Autodesk Inventor part; units mm, degrees
ref_plane "YZ Plane" through (0, 0, 0) normal (1, 0, 0) x (0, 1, 0)
ref_plane "XZ Plane" through (0, 0, 0) normal (0, 1, 0) x (-1, 0, 0)
ref_plane "XY Plane" through (0, 0, 0) normal (0, 0, 1) x (1, 0, 0)
sketch "Sketch1" plane through (0, 0, 0) normal (0, 1, 0) x (-1, 0, 0)
  line L0 (0, 0) -> (50, 0)
  line L1 (50, 0) -> (50, -50)
  line L2 (50, -50) -> (0, -50)
  line L3 (0, -50) -> (0, 0)
  dimension "d0" = 50
  dimension "d1" = 50
extrude "Extrusion1" add sketch "Sketch1" along normal blind 20
sketch "Sketch2" plane through (0, 0, 0) normal (1, 0, 0) x (0, 0, -1)
  line L0 (0, 20) -> (50, 20)
  line L1 (0, 0) -> (0, 20)
  line L2 (50, 0) -> (50, 20)
  point P0 (10, 10)
  point P1 (40, 10)
  dimension "d4" = 10
  dimension "d5" = 10
  dimension "d6" = 10
  dimension "d7" = 10
hole "Hole1" at (0, 10, -10) at (0, 10, -40) direction (-1, 0, 0) diameter 12 depth 50 tip angle 118
sketch "Sketch3" plane through (0, 20, 0) normal (0, 1, 0) x (1, 0, 0)
  line L0 (-50, 0) -> (-50, 50)
  line L1 (0, 50) -> (-50, 50)
  point P0 (0, 0)
  point P1 (-25, 25)
  dimension "d15" = 25
  dimension "d16" = 25
hole "Hole2" at (-25, 20, -25) direction (0, -1, 0) diameter 12 depth 50 tip angle 118
properties part number "Extruder mount top"
Check sheet for the modelled part. Datum: model origin and axes. Units: mm. Give positions to 0.01 mm unless a question says otherwise; leave off trailing zeros. Write each loop counter-clockwise with the first axis right and the second up, starting at its lowest first coordinate (ties: lowest second). Pieces come first, ordered by that corner, then holes.
Item 1: Cross-section at D-D (y = 1.5). Enter the section's corners in (x, z).
Item 2: Cross-section at B-B (y = 10). Enter the section's corners in (x, z), and give its area (3 significant figures).
Item 3: Scan lines: L1, parallel to Z at x = -34, y = 10; L2, parallel to Y at x = -21, z = -10; L3, parallel to Z at x = -25, y = 13. Record each from-to range of solid material in increasing order.
Item 4: Cross-section at A-A (z = -40). Enter the section's corners in (x, y), and give its area (3 significant figures).
Item 5: Draft check along Z on faces 1 (the face through (-25, 10, 0)), 2 (the face through (-25.35, 5.94, -35.58)), 3 (the face through (-25, 10, -50)). Enter one of: released by +Z, released by -Z, zero draft, split by the parting line, or undercut.
Item 6: Cross-section at C-C (x = -29.5). Enter the section's corners in (y, z), and give its area (3 significant figures).
Report:
1. outline: (-50, -50) - (0, -50) - (0, 0) - (-50, 0) - close; hole circle Ø12 at (-25, -25)
2. outline: (-50, -50) - (0, -50) - (0, -46) - (-50, -46) - close; (-50, -34) - (0, -34) - (0, -16) - (-50, -16) - close; (-50, -4) - (0, -4) - (0, 0) - (-50, 0) - close; hole circle Ø12 at (-25, -25)
2. area: 1,190 mm2
3. L1: z = -50 to -46, -34 to -16, -4 to 0
3. L2: y = 0 to 4, 16 to 20
3. L3: z = -50 to -45.2, -34.8 to -31, -19 to -15.2, -4.8 to 0
4. outline: (-50, 0) - (0, 0) - (0, 4) - (-50, 4) - close; (-50, 16) - (0, 16) - (0, 20) - (-50, 20) - close
4. area: 400 mm2
5. face 1: released by +Z
5. face 2: undercut
5. face 3: released by -Z
6. outline: (0, -50) - (20, -50) - (20, -28.97) - (0, -28.97) - close; (0, -21.03) - (20, -21.03) - (20, 0) - (0, 0) - close; hole circle Ø12 at (10, -40); hole circle Ø12 at (10, -10)
6. area: 615 mm2
